Geometry: see drawing. Coordinates: mm, zero at the bounding-box minimum. A direction names the side the tool comes from. Coordinates: 2 decimals unless noted, no trailing zeros. Loops run counter-clockwise (first coordinate to the right, second up) from the corner with the lowest first, then second, coordinate; pieces in that order, holes last. Notation, with made-up numbers: (88.25, 68) -> (147.25, 68) arc R22 ccw to (147.25, 85) -> close; hole circle Ø1 at (71, -25). An arc over 180 degrees is marked (long way). Answer as a JSON object with one key per item and string values.
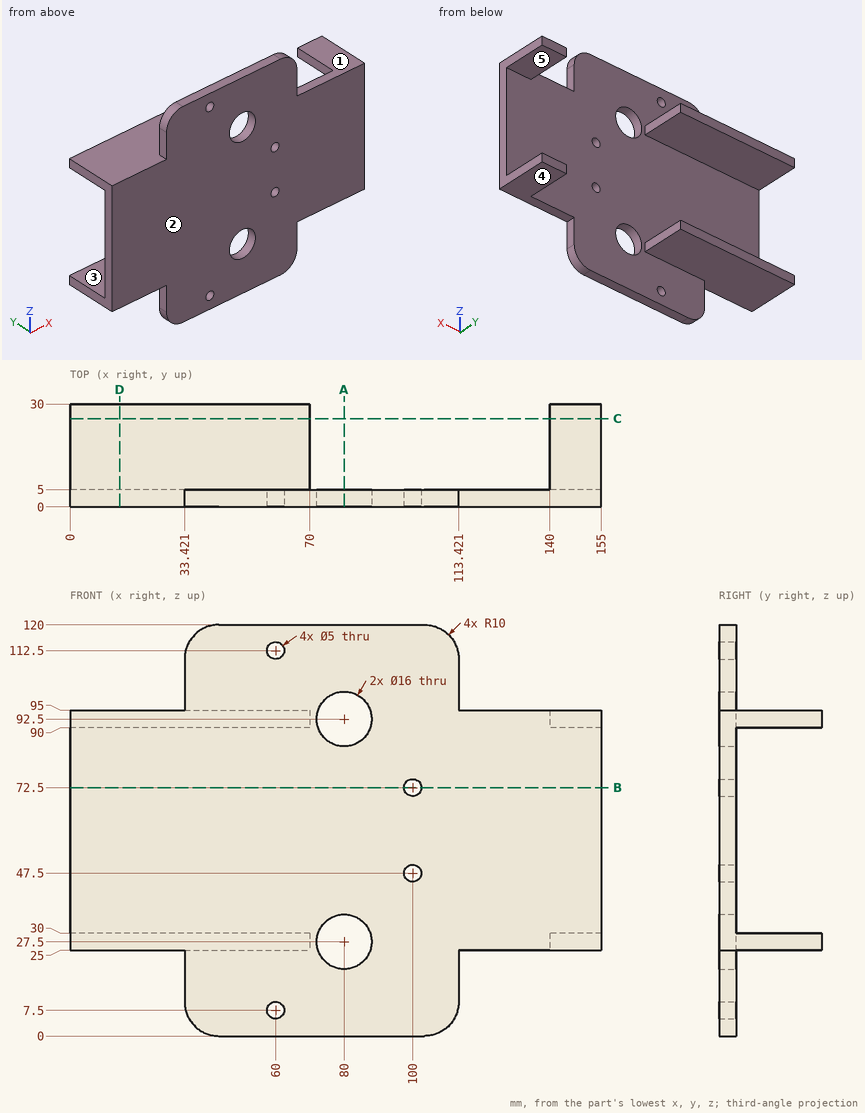
1. Section query B-B (z = 72.5). Return loops of the section in (x, y), plus the area to 3 significant figures.
Reply:
{"outline": "(0, 0) -> (97.5, 0) -> (97.5, 5) -> (0, 5) -> close; (102.5, 0) -> (155, 0) -> (155, 5) -> (102.5, 5) -> close", "area": "750 mm2"}
2. Section query D-D (x = 14.5). Return loops of the section in (y, z), plus the area to 3 significant figures.
Reply:
{"outline": "(0, 25) -> (30, 25) -> (30, 30) -> (5, 30) -> (5, 90) -> (30, 90) -> (30, 95) -> (0, 95) -> close", "area": "600 mm2"}
3. Line query: line 1 along Z through (x, y) = (80, 2.65); line 2 along X through (y, z) = (2.25, 92.5); line 3 along Z through (x, y) = (60, 3.55). Output: solid intervals per line, ascending.
Reply:
{"line 1": "z = 0 to 19.5, 35.5 to 84.5, 100.5 to 120", "line 2": "x = 0 to 72, 88 to 155", "line 3": "z = 0 to 5, 10 to 110, 115 to 120"}
4. Pin query (flat end, axial travel): P1, Ø6, axis at x = 79, y = 6, coming from the +Z side; P2, Ø6, axis at x = 60, z = 112.5, coming from the +Y side; P3, Ø15, axis at x = 137.5, y = 19.5, coming from the +Z side; P4, Ø12.5, axis at x = 33.5, y = 19, coming from the -Z side. Return the tip coordinate at first contact, or that it passes through.
Reply:
{"P1": "stops at z = 120", "P2": "stops at y = 5", "P3": "stops at z = 95", "P4": "stops at z = 25"}
5. Section query C-C (y = 25.75). Return loops of the section in (x, z).
Reply:
{"outline": "(0, 25) -> (70, 25) -> (70, 30) -> (0, 30) -> close; (0, 90) -> (70, 90) -> (70, 95) -> (0, 95) -> close; (140, 25) -> (155, 25) -> (155, 30) -> (140, 30) -> close; (140, 90) -> (155, 90) -> (155, 95) -> (140, 95) -> close"}
6. Mould query, pull axis Z, two halves, no side actions, for the marked faces 1, 2 and 3. Classes: pulls with the +Z half, pulls with the -Z half, needs draft (parallel to the pull), parting line crosses it, or undercut.
Reply:
{"face 1": "pulls with the +Z half", "face 2": "needs draft", "face 3": "undercut"}
7. Access query for the marked faces 4 and 5. Directions: +Z, -Z, +X, -X, +Y, -Y. A direction counts if a zero-diameter tool reaches every point of the face in a straight line with its end or side. Return the directions, or none.
Reply:
{"face 4": "-Z, +X, +Y, -Y", "face 5": "+X, -X, +Y"}
8. Section query A-A (x = 80). Return loops of the section in (y, z).
Reply:
{"outline": "(0, 0) -> (5, 0) -> (5, 19.5) -> (0, 19.5) -> close; (0, 35.5) -> (5, 35.5) -> (5, 84.5) -> (0, 84.5) -> close; (0, 100.5) -> (5, 100.5) -> (5, 120) -> (0, 120) -> close"}
